Can you work these out from the model? Positions are in its coordinate system, mm. Round coordinates to 2 decimals unless told otherwise and drop trailing zeros. Write each loop counter-clockwise with the first axis right and the second up, starting at its lowest first coordinate (ties: lowest second). Pieces come first, ordered by that corner, then holes. Notation, with made-up numbers: M -28.75,71 L -18.75,71 A33 ccw -18.75,107 Z; hole C -9,8.25 d11. An arc over 180 degrees is marked long. Answer in a Markdown table with one row per item. Add a question column.
(1) I'm going to push flat-ended pins straight in: pin 1 (2 mm diameter, centred on x = 1, z = -55.5, fed in from -Y); pin 2 (1.5 mm diameter, centred on x = 3, z = 1.5, fed in from +Y); pin 3 (1 mm diameter, centred on x = -1.5, z = -4.5, fed in from -Y); pin 4 (1.5 mm diameter, centred on x = -2, z = -28, fed in from +Y). Where does each tip first touch, or does it pass through?
(2) Suppose I cut it at A-A, the plane z = 83. Write out the boundary of the cut face in (x, y).
(3) If I drill on probe 1 along Y at (x, z) = (0, 109.7); probe 2 along Y at (x, z) = (0, 115.75); probe 3 along Z at (x, y) = (-1, 1), over which ranges is the centre line in solid material (lowest first)?
from build123d import *

# Parameters (mm, degrees)
SKETCH1_R                       = 3.96875
BOSS_EXTRUDE1_DEPTH             = 117.475
F_6_32_TAPPED_HOLE1_D           = 2.7051
F_6_32_TAPPED_HOLE1_DEPTH       = 9.398
F_6_32_TAPPED_HOLE1_CBORE_D     = 3.5052
F_6_32_TAPPED_HOLE1_CBORE_DEPTH = 7.112
F_6_32_TAPPED_HOLE1_TIP         = 0.81269403
F_6_32_TAPPED_HOLE2_D           = 2.7051
F_6_32_TAPPED_HOLE2_DEPTH       = 9.398
F_6_32_TAPPED_HOLE2_CBORE_D     = 3.5052
F_6_32_TAPPED_HOLE2_CBORE_DEPTH = 7.112
F_6_32_TAPPED_HOLE2_TIP         = 0.81269403


with BuildPart() as part:
    # Sketch1 → Boss-Extrude1 (new, symmetric)
    with BuildSketch(Plane.XY):
        Circle(SKETCH1_R)
    extrude(amount=BOSS_EXTRUDE1_DEPTH, both=True)

    # #6-32 Tapped Hole1
    with Locations(Plane(origin=(0, 0, -117.475), x_dir=(-1, 0, 0), z_dir=(0, 0, -1))):
        with Locations((0, 0)):
            CounterBoreHole(F_6_32_TAPPED_HOLE1_D / 2, F_6_32_TAPPED_HOLE1_CBORE_D / 2, F_6_32_TAPPED_HOLE1_CBORE_DEPTH, depth=F_6_32_TAPPED_HOLE1_DEPTH)
            with Locations((0, 0, -(F_6_32_TAPPED_HOLE1_DEPTH + F_6_32_TAPPED_HOLE1_TIP / 2))):  # 118° drill point
                Cone(0, F_6_32_TAPPED_HOLE1_D / 2, F_6_32_TAPPED_HOLE1_TIP, mode=Mode.SUBTRACT)

    # #6-32 Tapped Hole2
    with Locations(Plane.XY.offset(117.475)):
        with Locations((0, 0)):
            CounterBoreHole(F_6_32_TAPPED_HOLE2_D / 2, F_6_32_TAPPED_HOLE2_CBORE_D / 2, F_6_32_TAPPED_HOLE2_CBORE_DEPTH, depth=F_6_32_TAPPED_HOLE2_DEPTH)
            with Locations((0, 0, -(F_6_32_TAPPED_HOLE2_DEPTH + F_6_32_TAPPED_HOLE2_TIP / 2))):  # 118° drill point
                Cone(0, F_6_32_TAPPED_HOLE2_D / 2, F_6_32_TAPPED_HOLE2_TIP, mode=Mode.SUBTRACT)


solid = part.part
Calculated:
| question | item | result |
|---|---|---|
| 1 | pin 1 | y = -3.97 |
| 1 | pin 2 | y = 3.27 |
| 1 | pin 3 | y = -3.84 |
| 1 | pin 4 | y = 3.77 |
| 2 | outline | C 0,0 d7.94 |
| 3 | probe 1 | -3.97 to -1.35, 1.35 to 3.97 |
| 3 | probe 2 | -3.97 to -1.75, 1.75 to 3.97 |
| 3 | probe 3 | -110.36 to 110.36 |
